Geometry: final body of the model. Coordinates: model frame, mm. Face numbers are marked on the shaded views. A direction names the side the tool comes from. Round coordinates to 2 decimals unless told otherwise and drop trailing zeros. Loops run counter-clockwise (first coordinate to the right, second up) from the corner with the lowest first, then second, coordinate; pieces in that order, holes last. Notation, with made-up numbers: M -17,83.5 L 10,83.5 A24 cw 10,101.5 Z; hole C 75,38 d6. An arc over 180 degrees is marked long. Answer as a JSON object with one key per item and string values.
from build123d import *

# Parameters (mm, degrees)
F1_DEPTH = 21
F2_R     = 12.2992849538
F3_DEPTH = 4
F5_DEPTH = 3.6


# Not quite as in the source:
# - a pattern or mirror of a feature is missing from the dataset's text; its kind, count and spacing are read off the source's solid


with BuildPart() as f1:
    # F0 (on Top) → F1 (new body, symmetric)
    with BuildSketch(Plane.XY):
        Polygon((-40, 4), (-40, 0), (0, 0), (0, 40), (-4, 40), (-4, 4), align=None)
    extrude(amount=F1_DEPTH, both=True)

    # F2 (on face) → F3 (cut, through all)
    with BuildSketch(Plane(origin=(-4, 0, 0), x_dir=(0, -1, 0), z_dir=(-1, 0, 0))):
        with Locations((-22, 0)):
            Circle(F2_R)
    extrude(amount=-F3_DEPTH, mode=Mode.SUBTRACT)

    # F4 (on face) → F5 (join)
    with BuildSketch(Plane.XY.offset(21)):
        Polygon((-4, 40), (-40, 4), (-4, 4), align=None)
    f5 = extrude(amount=-F5_DEPTH)

    # F5_copies: F5 across plane
    add(f5.mirror(Plane(origin=(0, 0, 0), x_dir=(-1, 0, 0), z_dir=(0, 0, -1))))


solid = f1.part
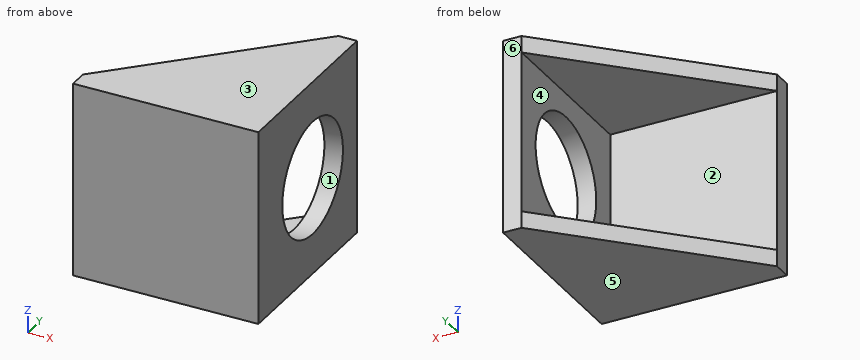
1) Ray query, line 1 (Z direction, x = -2.3, y = 22); line 2 (Z direction, x = -8.5, y = 14); line 3 (Y direction, x = -24.5, z = -3.5). Return the intervals inside material, ascending.
Results:
{"line 1": "-21 to -12.3, 12.3 to 21", "line 2": "-21 to -17.4, 17.4 to 21", "line 3": "0 to 4"}
2) Section query D-D (y = 37.5). Return the cut outline in (x, z), and give its area (3 significant figures).
Results:
{"outline": "M -6.5,-21 L 0,-21 L 0,21 L -6.5,21 L -6.5,17.4 L -4,17.4 L -4,-17.4 L -6.5,-17.4 Z", "area": "186 mm2"}
3) Pin query (flat end, axial travel): P1, Ø17.5, axis at x = -16.5, z = -1, coming from the +Y side; P2, Ø17.5, axis at y = 28.5, z = 5, coming from the -X side; P3, Ø5, axis at y = 10, z = -12, coming from the +X side. Return the tip coordinate at first contact, or that it passes through.
Results:
{"P1": "y = 4", "P2": "x = -4", "P3": "x = 0"}
4) Pull-direction query (Z, two-part tool) for the marked faces 3, 4, 5 and 6; classes: +Z half, -Z half, draft (parallel to the pull), parting line (faces both ways), or undercut.
Results:
{"face 3": "+Z half", "face 4": "undercut", "face 5": "-Z half", "face 6": "draft"}
5) Section query B-B (y = 22). Return the cut outline in (x, z), and give its area (3 significant figures).
Results:
{"outline": "M -22,-21 L 0,-21 L 0,-12.3 L -4,-12.3 L -4,-17.4 L -22,-17.4 Z; M -22,17.4 L -4,17.4 L -4,12.3 L 0,12.3 L 0,21 L -22,21 Z", "area": "199 mm2"}
6) Section query C-C (x = -33). Return the cut outline in (y, z).
Results:
{"outline": "M 0,-21 L 11,-21 L 11,-17.4 L 4,-17.4 L 4,17.4 L 11,17.4 L 11,21 L 0,21 Z"}
7) Reachability of the marked faces 1 and 2 from +Z, -Z, +X, -X, +Y, -Y: full face, straight path, thin tool, end or side. Return the list, or none.
Results:
{"face 1": "+X, -X", "face 2": "-X, +Y"}
8) Section query A-A (z = 0). Return the cut outline in (x, y).
Results:
{"outline": "M -40,0 L 0,0 L 0,9.7 L -4,9.7 L -4,4 L -40,4 Z; M -4,34.3 L 0,34.3 L 0,40 L -4,40 Z"}
